from build123d import *

# Parameters (mm, degrees)
F1_DEPTH = 152.4


with BuildPart() as f1:
    # F0 (on Front) → F1 (new body, symmetric)
    with BuildSketch(Plane.XZ):
        with BuildLine():
            Line((231.817934, -225.382066), (273.135868, -225.382066))
            ThreePointArc((273.135868, -225.382066), (295.232066, -142.917934), (355.6, -82.55))
            Line((355.6, -82.55), (355.6, 0))
            Line((355.6, 0), (0, 0))
            Line((0, 0), (0, -336.55))
            Line((0, -336.55), (165.1, -336.55))
            Line((165.1, -336.55), (165.1, -349.25))
            Line((165.1, -349.25), (190.5, -349.25))
            Line((190.5, -349.25), (190.5, -266.7))
            Line((190.5, -266.7), (231.817934, -266.7))
            Line((231.817934, -266.7), (231.817934, -225.382066))
        make_face()
    extrude(amount=F1_DEPTH, both=True)


solid = f1.part
Input: part model. Units: mm. Frame: model coordinates. A direction names the side the tool comes from. Round coordinates to 2 decimals unless told otherwise and drop trailing zeros. Loops run counter-clockwise (first coordinate to the right, second up) from the corner with the lowest first, then second, coordinate; pieces in that order, holes last. Notation, with made-up numbers: M 87.5,-1.75 L 119.5,-1.75 A21 cw 119.5,35.25 Z; hole C 47.25,9 d10. An arc over 180 degrees is marked long. Answer as CSV lines item,"result". Start each with the question number.
(1) First-contact query: pin 1 (10 mm diameter, centred on y = -40.5, z = -340, fed in from -X); pin 2 (20.5 mm diameter, centred on y = -22, z = -253.5, fed in from +X); pin 3 (2 mm diameter, centred on x = 310, y = -53.5, fed in from -Z); pin 4 (25 mm diameter, centred on y = -53.5, z = -310.5, fed in from +X). Flat tips, straight axial feed; report the tip coordinate or a pass-through.
(2) Reachability of faces 4 (the flat face through (81, -2, -336.55)), 5 (the flat face through (252, -2, -225.382)), 6 (the flat face through (355.6, -2, -42)) from +Z, -Z, +X, -X, +Y, -Y: full face, straight path, thin tool, end or side. Return the list, or none.
(3) Section B-B, the plane z = -313. Output: boundary loops of the cut face in (x, y).
(4) Section A-A, the plane y = -16. Output: boundary loops of the cut face in (x, z), plus the area to 3 significant figures.
(5) Line query: line 1 (Z direction, x = 252.5, y = -80.5); line 2 (Z direction, x = 133, y = -133); line 3 (X direction, y = 118.5, z = -230.5). Output: solid intervals per line, ascending. Write a range as [from, to].
(6) Draft query along Y for faces 1 (the flat face through (136, 152.4, -133)), 2 (the flat face through (136, -152.4, -133)), 3 (the flat face through (178, -2, -349.25)). Return one class per face: released by +Y, released by -Y, zero draft, split by the parting line, or undercut.
(7) Section C-C, the plane x = 115.5. Output: boundary loops of the cut face in (y, z).
Values found:
1,pin 1,"stops at x = 0"
1,pin 2,"stops at x = 231.82"
1,pin 3,"stops at z = -122.7"
1,pin 4,"stops at x = 190.5"
2,face 4,"-Z, -X, +Y, -Y"
2,face 5,"-Z, +X, +Y, -Y"
2,face 6,"+Z, -Z, +X, +Y, -Y"
3,outline,"M 0,-152.4 L 190.5,-152.4 L 190.5,152.4 L 0,152.4 Z"
4,outline,"M 0,-336.55 L 165.1,-336.55 L 165.1,-349.25 L 190.5,-349.25 L 190.5,-266.7 L 231.82,-266.7 L 231.82,-225.38 L 273.14,-225.38 A164.93 cw 355.6,-82.55 L 355.6,0 L 0,0 Z"
4,area,"95,000 mm²"
5,line 1,"z = [-225.38, 0]"
5,line 2,"z = [-336.55, 0]"
5,line 3,"x = [0, 231.82]"
6,face 1,"released by +Y"
6,face 2,"released by -Y"
6,face 3,"zero draft"
7,outline,"M -152.4,-336.55 L 152.4,-336.55 L 152.4,0 L -152.4,0 Z"
